```python
from build123d import *

# Parameters (mm, degrees)
F0_R     = 15.875
F1_DEPTH = 63.5
F2_W     = 32.258
F2_H     = 101.6
F3_DEPTH = 25.4
F4_R     = 16.129
F5_DEPTH = 76.2


with BuildPart() as f1:
    # F0 (on Front) → F1 (new body)
    with BuildSketch(Plane.XZ):
        Circle(F0_R)
    extrude(amount=F1_DEPTH)

    # F2 (on Front) → F3 (join)
    with BuildSketch(Plane.XZ):
        with Locations((0.108262, 33.494265)):
            Rectangle(F2_W, F2_H)
    extrude(amount=F3_DEPTH)

    # F4 (on Front) → F5 (join)
    with BuildSketch(Plane.XZ):
        with Locations((0.137554, 67.053316)):
            Circle(F4_R)
    extrude(amount=-F5_DEPTH)


solid = f1.part
```
CAD build for the part. Positions are in the model's coordinates, mm. A direction names the side the tool comes from. Give positions to 0.01 mm unless a question says otherwise; leave off trailing zeros. Loops run counter-clockwise (first coordinate to the right, second up) from the corner with the lowest first, then second, coordinate; pieces in that order, holes last. Notation, with made-up numbers: (65, 15.25) - (117, 15.25) arc R30 cw to (117, 46.25) - close; hole circle Ø3 at (1.25, 85.25). An arc over 180 degrees is marked (long way). Put each result on its own line as item: value.
Q1. Flat gauge pins, fed straight in: pin 1 (2 mm diameter, centred on x = -2.5, y = -42, fed in from +Z); pin 2 (16 mm diameter, centred on x = -2.5, z = 23, fed in from +Y); pin 3 (5 mm diameter, centred on x = 4.5, y = -38.5, fed in from -Z). Where does each tip first touch, or does it go through?
Filled in:
pin 1: stops at z = 15.8
pin 2: stops at y = 0
pin 3: stops at z = -15.75
Q2. Slice it at B-B (x = 12). Give the cut face in (y, z).
Filled in:
outline: (-63.5, -10.39) - (-25.4, -10.39) - (-25.4, -17.31) - (0, -17.31) - (0, 56.13) - (76.2, 56.13) - (76.2, 77.98) - (0, 77.98) - (0, 84.29) - (-25.4, 84.29) - (-25.4, 10.39) - (-63.5, 10.39) - close
Q3. Probe line 1 along Z through (x, y) = (0.5, 35); line 2 along Y through (x, z) = (-5.5, 49.5); line 3 along Z through (x, y) = (0.5, -35). List the from-to ranges inside material, lowest first.
Filled in:
line 1: z = 50.93 to 83.18
line 2: y = -25.4 to 0
line 3: z = -15.87 to 15.87
Q4. Slice it at A-A (z = 0). Give the cut face in (x, y) (3 decimals), plus the area to 3 significant figures.
Filled in:
outline: (-16.021, -25.4) - (-15.875, -25.4) - (-15.875, -63.5) - (15.875, -63.5) - (15.875, -25.4) - (16.237, -25.4) - (16.237, 0) - (-16.021, 0) - close
area: 2,030 mm²
Q5. Slice it at D-D (z = 29.5). Give the cut face in (x, y).
Filled in:
outline: (-16.02, -25.4) - (16.24, -25.4) - (16.24, 0) - (-16.02, 0) - close
Q6. Tool access for faces 1 (the face through (-3.441, -44.183, -15.497)), 2 (the face through (0, -63.5, 0)), 3 (the face through (-3.36, 37.57, 51.31)): list every direction of +Z, -Z, +X, -X, +Y, -Y with a clear straight run to the whole face (end or side of a thin tool).
Filled in:
face 1: -Y
face 2: +Z, -Z, +X, -X, -Y
face 3: +Y
Q7. Slice it at C-C (y = 34). Give the cut face in (x, z), plus the area to 3 significant figures.
Filled in:
outline: circle Ø32.26 at (0.14, 67.05)
area: 817 mm²
